Model file for the job. Use its own axes, mm. A direction names the side the tool comes from. Round coordinates to 2 decimals unless told otherwise and drop trailing zeros. Loops run counter-clockwise (first coordinate to the right, second up) from the corner with the lowest first, then second, coordinate; pieces in that order, holes last. Notation, with made-up numbers: (21, 79.25) -> (53, 79.25) arc R30 cw to (53, 118.25) -> close; hole circle Ø11 at (69, -13). An arc over 180 degrees is marked (long way). Use a Markdown table: item, result.
Autodesk Inventor part; units mm, degrees
ref_plane "Work Plane2" through (-30, -3, 7.5) normal (0, 1, 0) x (1, 0, 0)
ref_plane "YZ Plane" through (0, 0, 0) normal (1, 0, 0) x (0, 1, 0)
ref_plane "XZ Plane" through (0, 0, 0) normal (0, 1, 0) x (-1, 0, 0)
sketch "Sketch1" plane through (0, 0, 0) normal (0, 0, 1) x (1, 0, 0)
  circle A0 centre (0, 0) radius 3
  circle A1 centre (0, 0) radius 7.5
  line L0 (0, 7.5) -> (-5, 7.5)
  line L1 (-5, 7.5) -> (-5, -7.5)
  line L2 (-5, -7.5) -> (0, -7.5)
  dimension "d30" = 5
extrude "Extrusion2" add sketch "Sketch1" along normal blind 3 contours A1 L1 | A1 L1 L0 | L2 L1 A1 picked at (-4.3333, 0)
sketch "Sketch5" plane through (-5, -7.5, 0) normal (-1, 0, 0) x (0, 0, 1)
  line L0 (0, 15) -> (0, 0)
  line L1 (0, 0) -> (3, 0)
  line L2 (3, 15) -> (3, 0)
  line L3 (0, 15) -> (3, 15)
  point P0 (0, 7.5)
coil "Coil2" sketch "Sketch5" operation add axis through (-10, 0, 0) along (-1, 0, 0) pitch 100 turns 0.25 hand left
ref_plane "Work Plane2" through (-30, -3, 7.5) normal (0, 1, 0) x (1, 0, 0)
sketch "Sketch6" plane through (-30, -3, 7.5) normal (0, 1, 0) x (1, 0, 0)
  arc A0 (-3.0474, 8.05) -> (-3.0474, 6.95) centre (-4, 7.5) ccw
  line L0 (-1.85, 8.05) -> (-1.85, 12.75)
  line L1 (-1.85, 2.25) -> (-1.85, 6.95)
  line L2 (-7.5, 1.4) -> (-2.7, 1.4)
  line L3 (-33.95, 6.95) -> (-33.95, 2.25)
  line L4 (-33.95, 12.75) -> (-33.95, 8.05)
  arc A1 (-32.7526, 6.95) -> (-32.7526, 8.05) centre (-31.8, 7.5) ccw
  line L5 (-33.95, 6.95) -> (-32.7526, 6.95)
  line L6 (-32.7526, 8.05) -> (-33.95, 8.05)
  line L7 (-28.3, 13.6) -> (-33.1, 13.6)
  line L8 (-2.7, 13.6) -> (-7.5, 13.6)
  arc A2 (-1.85, 12.75) -> (-2.7, 13.6) centre (-2.7, 12.75) ccw
  line L9 (-1.85, 8.05) -> (-3.0474, 8.05)
  line L10 (-3.0474, 6.95) -> (-1.85, 6.95)
  arc A3 (-2.7, 1.4) -> (-1.85, 2.25) centre (-2.7, 2.25) ccw
  arc A4 (-33.95, 2.25) -> (-33.1, 1.4) centre (-33.1, 2.25) ccw
  line L11 (-33.1, 1.4) -> (-28.3, 1.4)
  line L12 (-24.612, 1.4) -> (-28.3, 1.4)
  line L13 (-7.5, 1.4) -> (-21.488, 1.4)
  circle A5 centre (-23.05, 7.5) radius 2.25
  line L14 (-28.3, 13.6) -> (-24.612, 13.6)
  line L15 (-21.488, 13.6) -> (-7.5, 13.6)
  line L16 (-6.65, 2.25) -> (-6.65, 12.75)
  line L17 (-29.15, 12.75) -> (-29.15, 2.25)
  arc A6 (-29.15, 2.25) -> (-28.3, 1.4) centre (-28.3, 2.25) ccw
  arc A7 (-28.3, 13.6) -> (-29.15, 12.75) centre (-28.3, 12.75) ccw
  arc A8 (-33.1, 13.6) -> (-33.95, 12.75) centre (-33.1, 12.75) ccw
  arc A9 (-7.5, 1.4) -> (-6.65, 2.25) centre (-7.5, 2.25) ccw
  arc A10 (-6.65, 12.75) -> (-7.5, 13.6) centre (-7.5, 12.75) ccw
  line L18 (-24.612, 13.6) -> (-21.488, 13.6)
  line L19 (-21.488, 1.4) -> (-24.612, 1.4)
  line L20 (0, 0) -> (0, 15)
  line L21 (0, 15) -> (-4, 15)
  line L22 (-4, 15) -> (-4, 0)
  line L23 (-4, 0) -> (0, 0)
  line L24 (-4, 0) -> (-34, 0)
  line L25 (-34, 0) -> (-34, 15)
  line L26 (-34, 15) -> (-4, 15)
  circle A11 centre (-31.8, 7.5) radius 1.1
  circle A12 centre (-4, 7.5) radius 1.1
  point P0 (30, 7.5)
  point P1 (-32.7526, 8.05)
  point P2 (-3.0474, 8.05)
extrude "Extrusion3" add sketch "Sketch6" along normal blind 3 contours A0 L22 L8 A2 L0 L9 | L9 L0 A2 L8 L22 L21 L20 L23 L2 A3 L1 L10 A12 | A0 L22 L2 A9 L16 A10 L8 | A0 L10 L1 A3 L2 L22 | L8 L15 L18 L14 L7 A8 L4 L6 A11 L5 L3 A4 L11 L12 L19 L13 L2 L22 L24 L25 L26 | A7 L17 A6 L11 A4 L3 L5 A1 L6 L4 A8 L7
properties part number "tail"
Q1. Drill centre lines: L1, parallel to Z at x = -34, y = -1.05; L2, parallel to Z at x = -1, y = 6; L3, parallel to Y at x = -25, z = -3.75. Where is each one in solid material? Low to high. Write a range as from..to.
Results list:
| item | result |
|---|---|
| L1 | z = -7.5..-1.1, 1.1..7.5 |
| L2 | z = 0..3 |
| L3 | y = -4.37..-1.22 |
Q2. Flat gauge pins, fed straight in: pin 1 (2.5 mm diameter, centred on x = -45.5, y = -1.5, fed in from +Z); pin 2 (1.5 mm diameter, centred on x = -21, z = -2, fed in from +Y); pin 3 (5 mm diameter, centred on x = -22, z = -3, fed in from +Y); pin 4 (1 mm diameter, centred on x = -48.5, z = -5.5, fed in from -Y) (3 decimals). Where does each tip first touch, or does it go through?
Results list:
| item | result |
|---|---|
| pin 1 | stops at z = 7.5 |
| pin 2 | stops at y = -0.79 |
| pin 3 | stops at y = -0.27 |
| pin 4 | passes through |
Q3. Band-saw the part on B-B, the plane x = -47.5. Give the cut face in (y, z), plus the area to 3 significant figures.
Results list:
| item | result |
|---|---|
| outline | (-3, -7.5) -> (0, -7.5) -> (0, -6.1) -> (-3, -6.1) -> close; (-3, 6.1) -> (0, 6.1) -> (0, 7.5) -> (-3, 7.5) -> close |
| area | 8.40 mm² |
Q4. Pull direction Z, two halves, no side cores. Call faces 1 (the face through (-43, 0, 7)), 2 (the face through (-48, -2, -6.1)), 3 (the face through (-47, -2, 7.5)): released by +Z, released by -Z, zero draft, split by the parting line, or undercut.
Results list:
| item | result |
|---|---|
| face 1 | zero draft |
| face 2 | undercut |
| face 3 | released by +Z |
Q5. Tool access for faces 4 (the face through (-36.65, -2, 0)), 5 (the face through (3, 2, 0)), 6 (the face through (-3, -7.5, 1)), 7 (the face through (-43, -3, 7)): list every direction of +Z, -Z, +X, -X, +Y, -Y with a clear straight run to the whole face (end or side of a thin tool).
Results list:
| item | result |
|---|---|
| face 4 | +Y, -Y |
| face 5 | -Z, +X, +Y, -Y |
| face 6 | +Z, -Z, +X, -Y |
| face 7 | +Z, -Z, -X, -Y |
Q6. Band-saw the part on A-A, the plane x = -61.8. Give the cut face in (y, z), plus the area to 3 significant figures.
Results list:
| item | result |
|---|---|
| outline | (-3, -7.5) -> (0, -7.5) -> (0, -1.1) -> (-3, -1.1) -> close; (-3, 1.1) -> (0, 1.1) -> (0, 7.5) -> (-3, 7.5) -> close |
| area | 38.4 mm² |
